Autodesk Inventor part; units mm, degrees
ref_plane "YZ Plane" through (0, 0, 0) normal (1, 0, 0) x (0, 1, 0)
ref_plane "XZ Plane" through (0, 0, 0) normal (0, 1, 0) x (-1, 0, 0)
ref_plane "XY Plane" through (0, 0, 0) normal (0, 0, 1) x (1, 0, 0)
sketch "Sketch1" plane through (0, 0, 0) normal (0, 1, 0) x (-1, 0, 0)
  line L0 (-7.5, -3.5) -> (-7.5, 3.5)
  line L1 (-7.5, 3.5) -> (7.5, 3.5)
  line L2 (7.5, 3.5) -> (7.5, -3.5)
  line L3 (7.5, -3.5) -> (-7.5, -3.5)
  line L4 (-7.5, -3.5) -> (7.5, 3.5) construction
  line L5 (-7.5, 3.5) -> (7.5, -3.5) construction
  circle A0 centre (7.5, 0) radius 1.5
  circle A1 centre (-7.5, 0) radius 1.65
  line L6 (7.5, 3.5) -> (11, 3.5)
  line L7 (11, 3.5) -> (11, -3.5)
  line L8 (11, -3.5) -> (7.5, -3.5)
  line L9 (7.5, -3.5) -> (7.5, 3.5)
  line L10 (-7.5, 3.5) -> (-11, 3.5)
  line L11 (-11, 3.5) -> (-11, -3.5)
  line L12 (-11, -3.5) -> (-7.5, -3.5)
  line L13 (-7.5, -3.5) -> (-7.5, 3.5)
  point P0 (0, 0)
  dimension "d0" = 7
  dimension "d1" = 15
  dimension "d2" = 3
  dimension "d3" = 3.3
  dimension "d4" = 3.5
  dimension "d5" = 3.5
extrude "Extrusion1" add sketch "Sketch1" along normal blind 5 contours L12 L11 L10 L0 A1 | L0 A1 L1 L2 A0 L3 | L2 A0 L6 L7 L8
fillet "Fillet1" radius 3.5 4 edges at (-11, 2.5, -3.5) (-11, 2.5, 3.5) (11, 2.5, 3.5) (11, 2.5, -3.5)
sketch "Sketch2" plane through (0, 0, 0) normal (0, -1, 0) x (1, 0, 0)
  circle A0 centre (-7.5, 0) radius 1.5
  circle A1 centre (-7.5, 0) radius 3.5
  circle A2 centre (-7.5, 0) radius 1.65
  point P0 (0, 0)
  dimension "d9" = 3.3
extrude "Extrusion2" add sketch "Sketch2" along normal blind 5 contours A1 | A2
properties part number "m"
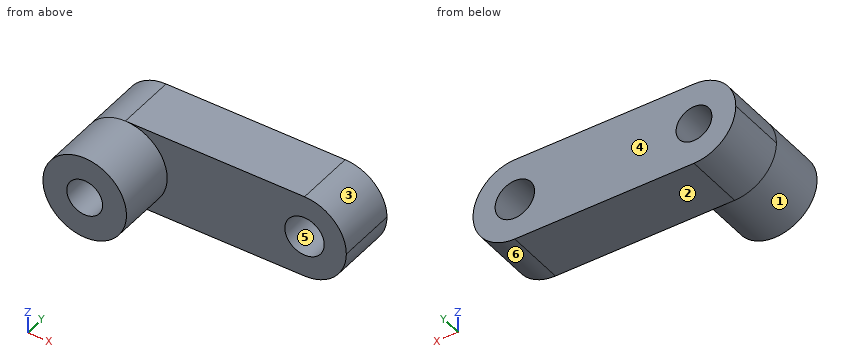
Model file for the job. Use its own axes, mm. Face numbers are marked on the shaded views. A direction names the side the tool comes from. Coordinates: 2 decimals unless noted, no trailing zeros. Write each loop counter-clockwise with the first axis right and the second up, starting at its lowest first coordinate (ties: lowest second). Pieces come first, ordered by that corner, then holes. Notation, with made-up numbers: (65, 60.25) - (124, 60.25) arc R17 ccw to (124, 84.25) - close; hole circle Ø9 at (35, 39.25). An arc over 180 degrees is marked (long way). One line per item, written item: value. Start each with the question number.
1. Slice it at A-A (y = 0.25). Count the separate pieces of the cut face and the enclosed holes in it, plus the area to 3 significant figures.
2. Flat gauge pins, fed straight in: pin 1 (3 mm diameter, centred on y = 1.5, z = 2.5, fed in from -X); pin 2 (2 mm diameter, centred on y = -2, z = 2.5, fed in from -X). Where does each tip first touch, or does it go through?
3. Mould opens along Z. For the marked faces 3, 4, 5 and 6 say: released by +Z, released by -Z, zero draft, split by the parting line, or undercut.
4. Probe line 1 (X direction, y = 3.1, z = 0); line 2 (Z direction, x = -7.5, y = 1.95); line 3 (X direction, y = -2.2, z = 0). List the from-to ranges inside material, lowest first. Write a range as from..to.
5. Slice it at B-B (z = -0.5). Write the cut outline in (x, y).
6. Tool access for the marked faces 1 and 2: list every direction of +Z, -Z, +X, -X, +Y, -Y with a clear straight run to the whole face (end or side of a thin tool).
7. Slice it at C-C (x = -4.75). Write the cut outline in (y, z), plus the area to 3 significant figures.
8. Slice it at D-D (y = -1.5). Write the cut outline in (x, z), plus the area to 3 significant figures.
Answers below:
1. separate pieces: 1
1. enclosed holes: 2
1. area: 128 mm^2
2. pin 1: stops at x = -10.85
2. pin 2: stops at x = -10.66
3. face 3: released by +Z
3. face 4: zero draft
3. face 5: undercut
3. face 6: released by -Z
4. line 1: x = -11..-9, -6..5.85, 9.15..11
4. line 2: z = -3.5..-1.5, 1.5..3.5
4. line 3: x = -11..-9, -6..-4
5. outline: (-10.96, -5) - (-8.91, -5) - (-8.91, 5) - (-10.96, 5) - close; (-6.09, -5) - (-4.04, -5) - (-4.04, 0) - (5.93, 0) - (5.93, 5) - (-6.09, 5) - close; (9.07, 0) - (10.96, 0) - (10.96, 5) - (9.07, 5) - close
6. face 1: -Y
6. face 2: -Z, +X, -X, +Y, -Y
7. outline: (-5, -2.17) - (0, -2.17) - (0, -3.5) - (5, -3.5) - (5, 3.5) - (0, 3.5) - (0, 2.17) - (-5, 2.17) - close
7. area: 56.7 mm^2
8. outline: circle Ø7 at (-7.5, 0); hole circle Ø3 at (-7.5, 0)
8. area: 31.4 mm^2
